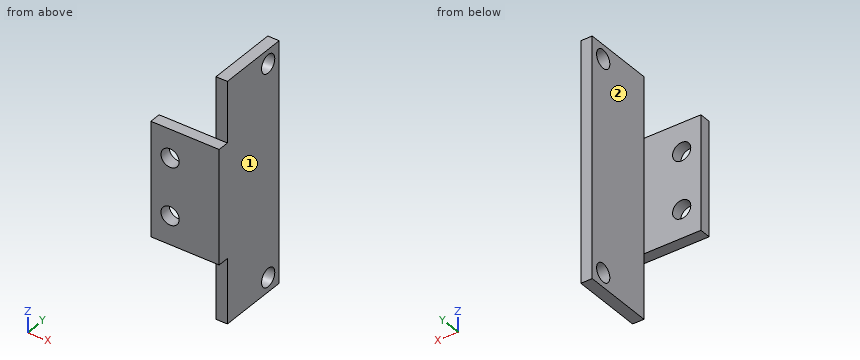
from build123d import *

# Parameters (mm, degrees)
SKETCH_1_W          = 12
SKETCH_1_H          = 20
EXTRUDE_1_DEPTH     = 2
SKETCH_2_W          = 2
SKETCH_2_H          = 11.337676179
SKETCH_2_H_2        = 20
SKETCH_2_H_3        = 10.662323821
EXTRUDE_3_DEPTH     = 20
SKETCH_5_R          = 1.6
SKETCH_5_W          = 42
SKETCH_5_H          = 7.454575948
CUT_EXTRUDE_1_DEPTH = 20
SKETCH_6_R          = 1.6
CUT_EXTRUDE_2_DEPTH = 10


with BuildPart() as part:
    # 草图1 → 凸台-拉伸1 (new body)
    with BuildSketch(Plane(origin=(0, 0, 0), x_dir=(1, 0, 0), z_dir=(0, 1, 0))):
        Rectangle(SKETCH_1_W, SKETCH_1_H)
    extrude(amount=EXTRUDE_1_DEPTH)

    # 草图2 → 凸台-拉伸3 (add)
    with BuildSketch(Plane(origin=(0, 2, 0), x_dir=(1, 0, 0), z_dir=(0, 1, 0))):
        with Locations((5, 15.66883809)):
            Rectangle(SKETCH_2_W, SKETCH_2_H)
        with Locations((5, 0)):
            Rectangle(SKETCH_2_W, SKETCH_2_H_2)
        with Locations((5, -15.331161911)):
            Rectangle(SKETCH_2_W, SKETCH_2_H_3)
    extrude(amount=EXTRUDE_3_DEPTH)

    # 草图5 → 切除-拉伸1 (cut)
    with BuildSketch(Plane(origin=(6, 0, 0), x_dir=(0, 0, -1), z_dir=(1, 0, 0))):
        with Locations((-18.162323821, 11.882323557)):
            Circle(SKETCH_5_R)
        with Locations((18.837676179, 11.882323557)):
            Circle(SKETCH_5_R)
        with Locations((0.337676179, 18.272712026)):
            Rectangle(SKETCH_5_W, SKETCH_5_H)
    extrude(amount=-CUT_EXTRUDE_1_DEPTH, mode=Mode.SUBTRACT)

    # 草图6 → 切除-拉伸2 (cut)
    with BuildSketch(Plane(origin=(0, 2, 0), x_dir=(1, 0, 0), z_dir=(0, 1, 0))):
        with Locations(Location((-2.620398145, 5, 0), (0, 0, 270))):
            Circle(SKETCH_6_R)
        with Locations(Location((-2.620398145, -5, 0), (0, 0, 270))):
            Circle(SKETCH_6_R)
    extrude(amount=-CUT_EXTRUDE_2_DEPTH, mode=Mode.SUBTRACT)


solid = part.part
Build history of the part. All positions in model axes, mm. Face numbers are marked on the shaded views. A direction names the side the tool comes from. Give positions to 0.01 mm unless a question says otherwise; leave off trailing zeros. Order: outer loops, then holes, each group sorted by start corner. A loop starts at its lowest first (then second) coordinate and runs counter-clockwise, first axis right, second up. Notation, with made-up numbers: M -3.5,-19 L 11.5,-19 A6 ccw 11.5,-14 Z; hole C 77,4 d2. An arc over 180 degrees is marked long. Put each result on its own line as item: value.
Item 1: Cut at D-D on y = 1.25. Write the cut outline in (x, z).
Results are:
outline: M -6,-10 L 6,-10 L 6,10 L -6,10 Z; hole C -2.62,-5 d3.2; hole C -2.62,5 d3.2
Item 2: Cut at C-C on x = 4.75. Write the cut outline in (y, z).
Results are:
outline: M 0,-10 L 2,-10 L 2,-21.34 L 14.55,-21.34 L 14.55,20.66 L 2,20.66 L 2,10 L 0,10 Z; hole C 11.88,-18.84 d3.2; hole C 11.88,18.16 d3.2
Item 3: Wall check: probe 1 along Y at (x, z) = (5.75, -19); probe 2 along X at (y, z) = (0.95, 5); probe 3 along X at (y, z) = (6.5, 10.5). Give the ranges that are in metal, low to high.
Results are:
probe 1: 2 to 10.29, 13.47 to 14.55
probe 2: -6 to -4.22, -1.02 to 6
probe 3: 4 to 6
Item 4: Drop flat-ended pins along their axis: pin 1 Ø2 at (x, z) = (4.5, -13.5) entering from -Y; pin 2 Ø4 at (y, z) = (11, -8) entering from -X; pin 3 Ø0.6 at (x, y) = (2.5, 0.5) entering from +Z. Give the stop position or say it passes through.
Results are:
pin 1: y = 2
pin 2: x = 4
pin 3: z = 10
Item 5: Cut at B-B on x = -3. Write the cut outline in (y, z).
Results are:
outline: M 0,-10 L 2,-10 L 2,-6.55 L 0,-6.55 Z; M 0,-3.45 L 2,-3.45 L 2,3.45 L 0,3.45 Z; M 0,6.55 L 2,6.55 L 2,10 L 0,10 Z
Item 6: Cut at A-A on z = 5. Write the cut outline in (x, y), then the cut area to 3 significant figures.
Results are:
outline: M -6,0 L -4.22,0 L -4.22,2 L -6,2 Z; M -1.02,0 L 6,0 L 6,14.55 L 4,14.55 L 4,2 L -1.02,2 Z
area: 42.7 mm2
Item 7: Which spindle directions (+Z, -Z, +X, -X, +Y, -Y) get a long thin tool onto all of the face, cutting with end or side? Do the marked faces 1 and 2. Say none if no direction does.
Results are:
face 1: +Z, -Z, +X, +Y, -Y
face 2: +Z, -Z, -X, +Y
